Autodesk Inventor part; units mm, degrees
ref_plane "YZ Plane" through (0, 0, 0) normal (1, 0, 0) x (0, 1, 0)
ref_plane "XZ Plane" through (0, 0, 0) normal (0, 1, 0) x (-1, 0, 0)
ref_plane "XY Plane" through (0, 0, 0) normal (0, 0, 1) x (1, 0, 0)
sketch "Boceto39" plane through (0, 0, 0) normal (0, 0, 1) x (1, 0, 0)
  line L0 (-1.27, 1.27) -> (1.27, 1.27)
  line L1 (1.27, 1.27) -> (1.27, -1.27)
  line L2 (1.27, -1.27) -> (-1.27, -1.27)
  line L3 (-1.27, -1.27) -> (-1.27, 1.27)
  point P0 (0, 0)
  point P1 (0, 1.27)
  point P2 (-1.27, 0)
  dimension "d373" = 2.54
extrude "Extrusión13" add sketch "Boceto39" along normal blind 8
sketch "Boceto40" plane through (0, 0, 8) normal (0, 0, 1) x (1, 0, 0)
  line L0 (-0.4, 0.4) -> (0.4, 0.4)
  line L1 (0.4, 0.4) -> (0.4, -0.4)
  line L2 (0.4, -0.4) -> (-0.4, -0.4)
  line L3 (-0.4, -0.4) -> (-0.4, 0.4)
  point P0 (0, 0)
  point P1 (0, 0.4)
  point P2 (-0.4, 0)
  dimension "d376" = 0.8
extrude "Extrusión14" cut sketch "Boceto40" against normal blind 8
chamfer "Chaflán5" distance 0.3 angle 45 4 edges at (0, 0.4, 8) (0.4, 0, 8) (0, -0.4, 8) (-0.4, 0, 8)
sketch "Boceto42" plane through (0, 0, 0) normal (0, 1, 0) x (-1, 0, 0)
  line L0 (-0.4, 7.7) -> (-0.4, 0) construction
  line L1 (0.4, 7.7) -> (0.4, 0) construction
  line L2 (-0.4, 0) -> (-0.3, 0)
  line L3 (-1.27, 0) -> (1.27, 0) construction
  line L4 (-0.3, -3) -> (-0.3, 0)
  line L5 (0.3, -3) -> (-0.3, -3)
  line L6 (0.3, -3) -> (0.3, 0)
  line L7 (0.3, 0) -> (0.4, 0)
  line L8 (0.4, 0) -> (0.4, 0.3601)
  line L9 (0.4, 0.3601) -> (-0.4, 0.3601)
  line L10 (-0.4, 0.3601) -> (-0.4, 0)
  point P0 (0, 0)
  point P1 (0, -3)
  point P2 (0, 0)
  dimension "d386" = 0.6
  dimension "d387" = 3
extrude "Extrusión16" add sketch "Boceto42" along normal mid plane 0.35
chamfer "Chaflán6" distance 0.15 angle 45 2 edges at (0.3, 0, -3) (-0.3, 0, -3)
properties part number "CON-HEM"
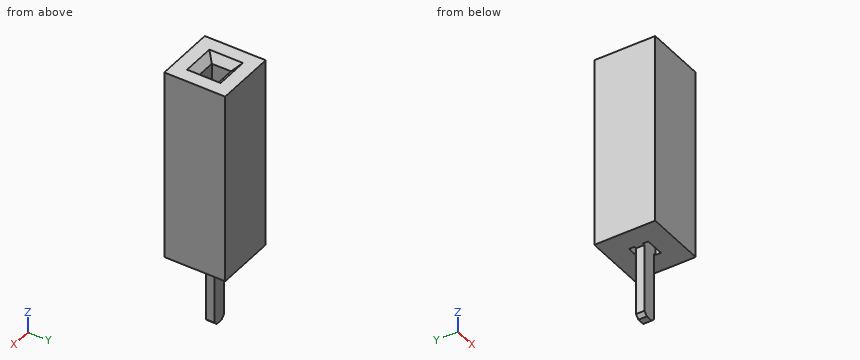
The listing builds one solid part. Answer for the finished solid, in the listing's coordinates (mm). Coordinates: 2 decimals unless noted, no trailing zeros. Loops run counter-clockwise (first coordinate to the right, second up) from the corner with the lowest first, then second, coordinate; pieces in that order, holes last. Notation, with made-up numbers: (37.25, -2) -> (56.25, -2) arc R30 cw to (56.25, 24) -> close; hole circle Ø10 at (89.25, -5). An arc over 180 degrees is marked (long way). Return JSON: item names as keys, results as strings. Group by question number.
(1) Given pin 1 Ø1 at (x, y) = (0.5, -1) entering from -Z, flat-ended and moving along its own axis, determine where the tip first touches the part or whether it passes through.
(2) A cutting plane is placed at C-C on y = 0. Write down the section's boundary in (x, z), and give its area (3 significant figures).
(3) Find the intervals of material crossed by probe 1 along X at (y, z) = (0.15, 6.5); probe 2 along Z at (x, y) = (-0.7, 0.9), in increasing order. Write a range as from..to.
(4) A cutting plane is placed at D-D on x = 0.5. Write down the section's boundary in (y, z), and give its area (3 significant figures).
(5) A cutting plane is placed at A-A on x = -0.05. Write down the section's boundary in (y, z) (3 decimals).
(6) A cutting plane is placed at B-B on z = 2. Write down the section's boundary in (x, y), and give its area (3 significant figures).
The answers:
{
 "1": {"pin 1": "stops at z = 0"},
 "2": {"outline": "(-1.27, 0) -> (-0.3, 0) -> (-0.3, -2.85) -> (-0.15, -3) -> (0.15, -3) -> (0.3, -2.85) -> (0.3, 0) -> (1.27, 0) -> (1.27, 8) -> (0.7, 8) -> (0.4, 7.7) -> (0.4, 0.36) -> (-0.4, 0.36) -> (-0.4, 7.7) -> (-0.7, 8) -> (-1.27, 8) -> close", "area": "15.9 mm^2"},
 "3": {"probe 1": "x = -1.27..-0.4, 0.4..1.27", "probe 2": "z = 0..8"},
 "4": {"outline": "(-1.27, 0) -> (1.27, 0) -> (1.27, 8) -> (0.7, 8) -> (0.5, 7.8) -> (-0.5, 7.8) -> (-0.7, 8) -> (-1.27, 8) -> close", "area": "20.1 mm^2"},
 "5": {"outline": "(-1.27, 0) -> (-0.4, 0) -> (-0.4, 7.7) -> (-0.7, 8) -> (-1.27, 8) -> close; (-0.175, -3) -> (0.175, -3) -> (0.175, 0.36) -> (-0.175, 0.36) -> close; (0.4, 0) -> (1.27, 0) -> (1.27, 8) -> (0.7, 8) -> (0.4, 7.7) -> close"},
 "6": {"outline": "(-1.27, -1.27) -> (1.27, -1.27) -> (1.27, 1.27) -> (-1.27, 1.27) -> close; hole (-0.4, -0.4) -> (0.4, -0.4) -> (0.4, 0.4) -> (-0.4, 0.4) -> close", "area": "5.81 mm^2"}
}
